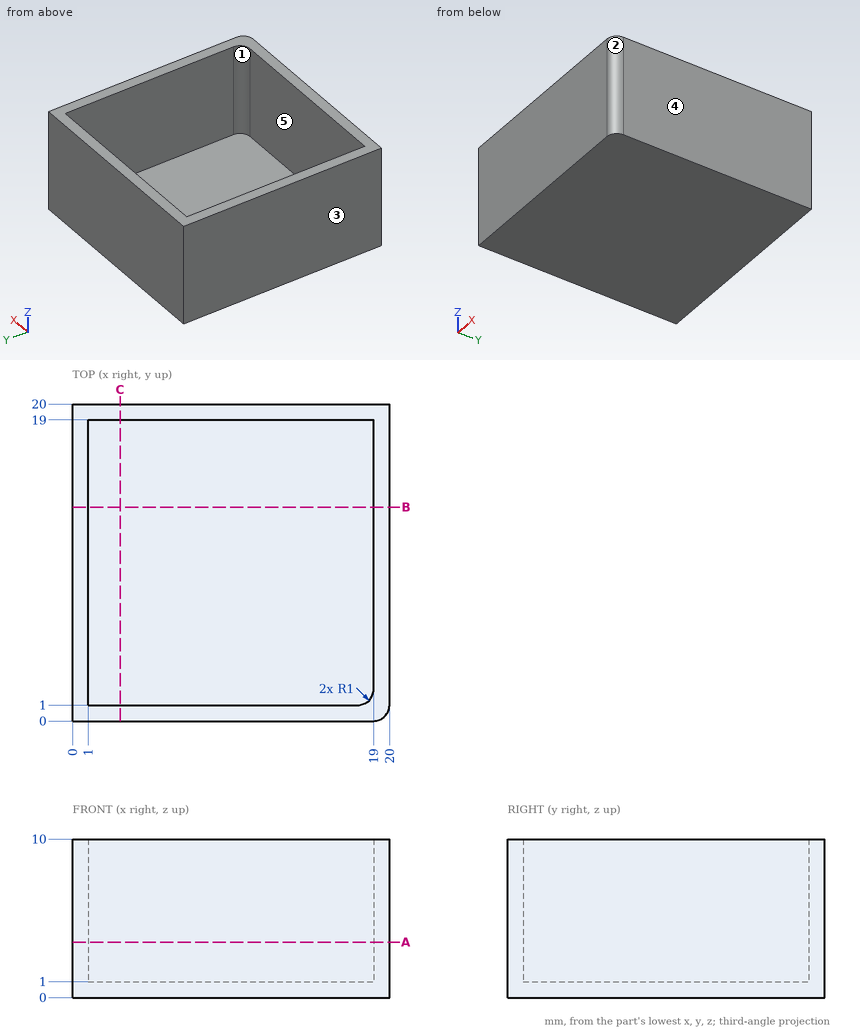
Answer from the drawing. Dimensions are ordinates in mm from the lowest x, y and z of the part. A direction names the side the tool comes from. Round coordinates to 2 decimals unless told otherwise and drop trailing zeros. Loops run counter-clockwise (first coordinate to the right, second up) from the corner with the lowest first, then second, coordinate; pieces in that order, holes last. Notation, with made-up numbers: (68, -10) - (127, -10) arc R11 ccw to (127, 10) - close; hole circle Ø3 at (-28.5, 20.5). An arc over 180 degrees is marked (long way). One line per item, written item: value.
Q1. The mould has two halves that part along Y. Classify the marked faces 1, 2 and 3: +Y half, -Y half, draft (parallel to the pull), parting line (faces both ways), or undercut.
Check values:
face 1: undercut
face 2: -Y half
face 3: draft
Q2. Find section A-A on z = 3.5. Give the vertices of the cut face in (x, y), and give its area (3 significant figures).
Check values:
outline: (0, 0) - (19, 0) arc R1 ccw to (20, 1) - (20, 20) - (0, 20) - close; hole (1, 1) - (18, 1) arc R1 ccw to (19, 2) - (19, 19) - (1, 19) - close
area: 76.0 mm2
Q3. For the marked faces 4 and 5, determine the directions among +Z, -Z, +X, -X, +Y, -Y from which every point of the face is accessible in a straight line to the end or side of a thin tool.
Check values:
face 4: +Z, -Z, +X, +Y, -Y
face 5: +Z
Q4. Find section B-B on y = 13.5. Give the vertices of the cut face in (x, z), and give its area (3 significant figures).
Check values:
outline: (0, 0) - (20, 0) - (20, 10) - (19, 10) - (19, 1) - (1, 1) - (1, 10) - (0, 10) - close
area: 38.0 mm2
Q5. Each of these flat-tipped pins is pushed along its axis until it touches: pin 1 Ø1.5 at (x, y) = (17.5, 11.5) entering from +Z; pin 2 Ø12 at (x, y) = (17.5, 2.5) entering from +Z. Where does it stop, or does it pass through?
Check values:
pin 1: z = 1
pin 2: z = 10
Q6. Straight lines are drawn through the part: probe 1 along Y at (x, z) = (1.75, 1.25); probe 2 along Z at (x, y) = (8.5, 16.25). For each, find the intervals that lie inside material, in ascending order.
Check values:
probe 1: 0 to 1, 19 to 20
probe 2: 0 to 1
